For this review, take the finished solid that the model builds, in its own axes (mm). A direction names the side the tool comes from. Round coordinates to 2 decimals unless told otherwise and drop trailing zeros. Loops run counter-clockwise (first coordinate to the right, second up) from the corner with the lowest first, then second, coordinate; pieces in that order, holes last. Notation, with made-up numbers: M -27.5,66 L 21.5,66 A9 cw 21.5,78 Z; hole C -19.75,86 d8. An arc over 180 degrees is marked long. One line per question, with ' | ' between items. Start each with the question number.
1) Mouldability with a two-part tool opening along Y and no side actions: class faces 3 (the face through (-97.62, -0.75, -175.27)), 4 (the face through (-55, -16, -74)), 5 (the face through (-66.373, -7.923, -79.231)) as pulls with the +Y half, pulls with the -Y half, needs draft (parallel to the pull), parting line crosses it, or undercut.
2) For pin 1 Ø4 at (y, z) = (-8.5, -84) entering from +X; pin 2 Ø1 at (x, y) = (-48, -14) entering from -Z; pin 3 Ø8 at (x, y) = (3, -5.5) entering from -Z; pin 4 Ø3 at (x, z) = (0, 0) entering from +Y, all flat-tipped, find the tip position at first contact; note any pin that passes through.
3) For probe 1 along Y at (x, z) = (10.5, 0.5); probe 2 along X at (y, z) = (-2, -0.5); probe 3 along X at (y, z) = (-12, 5), list the stretches that pass through material, from the lowest coordinate up. Write a range as from..to.
4) For faces 1 (the face through (-58.322, -7.923, -101.605)), 2 (the face through (0, -8, -3)), list the 3-axis set-ups (+Z, -Z, +X, -X, +Y, -Y) from which the entire face can be reached by the end or side of a thin tool; tool diameter is ignored.
5) We need section A-A (y = -10.5). Give the boundary of the cut face in (x, z), and give its area (3 significant figures).
```python
from build123d import *

# Parameters (mm, degrees)
F1_DEPTH     = 16
F2_DEPTH     = 8
F3_T1_DEPTH  = 28.5
F3_T3_DEPTH  = 176.25
F3_T5_DEPTH  = 206.25
F3_T8_ANGLE  = 113.8828315396
F3_T10_ANGLE = 205.3052563157
F3_T12_ANGLE = 301.0526480562
F3_T14_ANGLE = 87.1421031631
F3_T16_ANGLE = 90
F3_T18_ANGLE = 202.4999999088
F3_T20_ANGLE = 256.2183340246
F3_T22_ANGLE = 87.1421031631
F4_D         = 5


# Not quite as in the source:
# - a fillet or chamfer that OpenCascade refuses, or shapes differently, is made with other operations: its cross-section is extruded or revolved along the edge and cut away or added


with BuildPart() as f1:
    # F0 (on Front) → F1 (new body)
    with BuildSketch(Plane.XZ):
        Polygon((-25.3386959586, -21.9761344899), (-13.8581929877, 5.7402514855), (-28.6402655078, 11.8631864033), (-105.1769519809, -172.9127200989), (-90.3948794607, -179.0356550168), align=None)
        with BuildLine():
            Line((-28.6402655078, 11.8631864033), (-13.8581929877, 5.7402514855))
            ThreePointArc((-13.8581929877, 5.7402514855), (-8.3335534854, 12.4720441912), (2.39e-08, 15))
            ThreePointArc((2.39e-08, 15), (-8, 22.9999999881), (0, 31))
            ThreePointArc((0, 31), (-17.2226772236, 25.7755579814), (-28.6402655078, 11.8631864033))
        make_face()
        with BuildLine():
            ThreePointArc((-5.7402514855, -13.8581929877), (-13.8581929877, -5.7402514855), (-13.8581929877, 5.7402514855))
            Line((-13.8581929877, 5.7402514855), (-25.3386959586, -21.9761344899))
            ThreePointArc((-25.3386959586, -21.9761344899), (-17.2207544564, -13.8581929877), (-5.7402514855, -13.8581929877))
        make_face()
    extrude(amount=F1_DEPTH)

    # F0 (on Front) → F2 (join)
    with BuildSketch(Plane.XZ):
        with BuildLine():
            Line((0, 0), (-13.8581929877, 5.7402514855))
            ThreePointArc((-13.8581929877, 5.7402514855), (-13.8581929877, -5.7402514855), (-5.7402514855, -13.8581929877))
            Line((-5.7402514855, -13.8581929877), (0, 0))
        make_face()
        with BuildLine():
            ThreePointArc((2.39e-08, 15), (-8.3335534854, 12.4720441912), (-13.8581929877, 5.7402514855))
            Line((-13.8581929877, 5.7402514855), (0, 0))
            Line((0, 0), (-5.7402514855, -13.8581929877))
            ThreePointArc((-5.7402514855, -13.8581929877), (8.3335534953, -12.4720441845), (15, 0))
            ThreePointArc((15, 0), (10.6066017262, 10.6066017094), (2.39e-08, 15))
        make_face()
    extrude(amount=F2_DEPTH)

    # F3: fillet of radius 2.5 on 14 edges, made by hand

    # F3_s2 → F3_t1 (cut)
    with BuildSketch(Plane(origin=(-34.414512586, 0, 14.2549578556), x_dir=(0, 1, 0), z_dir=(0.9238795325, 0, -0.3826834324))):
        with BuildLine():
            ThreePointArc((-13.5, -200), (-15.267766953, -199.267766953), (-16, -197.5))
            Line((-16, -197.5), (-16, -200))
            Line((-16, -200), (-13.5, -200))
        make_face()
        with BuildLine():
            ThreePointArc((-2.5, -200), (-0.732233047, -199.267766953), (0, -197.5))
            Line((0, -197.5), (0, -200))
            Line((0, -200), (-2.5, -200))
        make_face()
    extrude(amount=F3_T1_DEPTH, mode=Mode.SUBTRACT)

    # F3_s4 → F3_t3 (cut)
    with BuildSketch(Plane(origin=(-78.9284579253, 0, -190.5501535805), x_dir=(0, 1, 0), z_dir=(0.3826834324, 0, 0.9238795325))):
        with BuildLine():
            ThreePointArc((-13.5, 15), (-15.267766953, 15.732233047), (-16, 17.5))
            Line((-16, 17.5), (-16, 15))
            Line((-16, 15), (-13.5, 15))
        make_face()
        with BuildLine():
            ThreePointArc((-2.5, 15), (-0.732233047, 15.732233047), (0, 17.5))
            Line((0, 17.5), (0, 15))
            Line((0, 15), (-2.5, 15))
        make_face()
    extrude(amount=F3_T3_DEPTH, mode=Mode.SUBTRACT)

    # F3_s6 → F3_t5 (cut)
    with BuildSketch(Plane(origin=(0, 0, 0), x_dir=(0, 1, 0), z_dir=(-0.3826834324, 0, -0.9238795325))):
        with BuildLine():
            ThreePointArc((-13.5, -31), (-15.267766953, -30.267766953), (-16, -28.5))
            Line((-16, -28.5), (-16, -31))
            Line((-16, -31), (-13.5, -31))
        make_face()
        with BuildLine():
            ThreePointArc((-2.5, -31), (-0.732233047, -30.267766953), (0, -28.5))
            Line((0, -28.5), (0, -31))
            Line((0, -31), (-2.5, -31))
        make_face()
    extrude(amount=F3_T5_DEPTH, mode=Mode.SUBTRACT)

    # F3_s7 → F3_t8 (revolve, cut)
    with BuildSketch(Plane(origin=(-11.480502971, 0, -27.7163859753), x_dir=(0, 1, 0), z_dir=(-0.3826834324, 0, -0.9238795325))):
        with BuildLine():
            ThreePointArc((-16, -17.5), (-15.267766953, -15.732233047), (-13.5, -15))
            Line((-13.5, -15), (-16, -15))
            Line((-16, -15), (-16, -17.5))
        make_face()
    revolve(axis=Axis((-11.480502971, -16, -27.7163859753), (0, 1, 0)), revolution_arc=F3_T8_ANGLE, mode=Mode.SUBTRACT)

    # F3_s9 → F3_t10 (revolve, cut)
    with BuildSketch(Plane(origin=(0, 0, 0), x_dir=(0, 1, 0), z_dir=(0.999700368, 0, 0.0244780336))):
        with BuildLine():
            ThreePointArc((-16, -17.5), (-15.267766953, -15.732233047), (-13.5, -15))
            Line((-13.5, -15), (-16, -15))
            Line((-16, -15), (-16, -17.5))
        make_face()
    revolve(axis=Axis((0, -16, 0), (0, 1, 0)), revolution_arc=F3_T10_ANGLE, mode=Mode.SUBTRACT)

    # F3_s11 → F3_t12 (revolve, cut)
    with BuildSketch(Plane(origin=(11.4998076678, 0, 11.4334898289), x_dir=(0, 1, 0), z_dir=(0.7091486068, 0, 0.7050590425))):
        with BuildLine():
            ThreePointArc((-16, 5.8104179571), (-15.267766953, 7.5781849101), (-13.5, 8.3104179571))
            Line((-13.5, 8.3104179571), (-16, 8.3104179571))
            Line((-16, 8.3104179571), (-16, 5.8104179571))
        make_face()
    revolve(axis=Axis((0, -16, 23), (0, 1, 0)), revolution_arc=F3_T12_ANGLE, mode=Mode.SUBTRACT)

    # F3_s13 → F3_t14 (revolve, cut)
    with BuildSketch(Plane(origin=(0, 0, 0), x_dir=(0, 1, 0), z_dir=(0.9418106956, 0, -0.3361437395))):
        with BuildLine():
            ThreePointArc((-16, 28.5), (-15.267766953, 30.267766953), (-13.5, 31))
            Line((-13.5, 31), (-16, 31))
            Line((-16, 31), (-16, 28.5))
        make_face()
    revolve(axis=Axis((0, -16, 0), (0, -1, 0)), revolution_arc=F3_T14_ANGLE, mode=Mode.SUBTRACT)

    # F3_s15 → F3_t16 (revolve, cut)
    with BuildSketch(Plane(origin=(-11.480502971, 0, -27.7163859753), x_dir=(0, 1, 0), z_dir=(-0.3826834324, 0, -0.9238795325))):
        with BuildLine():
            ThreePointArc((0, -17.5), (-0.732233047, -15.732233047), (-2.5, -15))
            Line((-2.5, -15), (0, -15))
            Line((0, -15), (0, -17.5))
        make_face()
    revolve(axis=Axis((-11.480502971, 0, -27.7163859753), (0, 1, 0)), revolution_arc=F3_T16_ANGLE, mode=Mode.SUBTRACT)

    # F3_s17 → F3_t18 (revolve, cut)
    with BuildSketch(Plane(origin=(0, 0, 0), x_dir=(0, 1, 0), z_dir=(-0.9238795325, 0, 0.3826834324))):
        with BuildLine():
            ThreePointArc((0, 12.5), (-0.732233047, 14.267766953), (-2.5, 15))
            Line((-2.5, 15), (0, 15))
            Line((0, 15), (0, 12.5))
        make_face()
    revolve(axis=Axis((0, 0, 0), (0, -1, 0)), revolution_arc=F3_T18_ANGLE, mode=Mode.SUBTRACT)

    # F3_s19 → F3_t20 (revolve, cut)
    with BuildSketch(Plane.YZ):
        with BuildLine():
            ThreePointArc((0, 12.5), (-0.732233047, 14.267766953), (-2.5, 15))
            Line((-2.5, 15), (0, 15))
            Line((0, 15), (0, 12.5))
        make_face()
    revolve(axis=Axis((0, 0, 23), (0, 1, 0)), revolution_arc=F3_T20_ANGLE, mode=Mode.SUBTRACT)

    # F3_s21 → F3_t22 (revolve, cut)
    with BuildSketch(Plane(origin=(0, 0, 0), x_dir=(0, 1, 0), z_dir=(0.9418106956, 0, -0.3361437395))):
        with BuildLine():
            ThreePointArc((0, 28.5), (-0.732233047, 30.267766953), (-2.5, 31))
            Line((-2.5, 31), (0, 31))
            Line((0, 31), (0, 28.5))
        make_face()
    revolve(axis=Axis((0, 0, 0), (0, -1, 0)), revolution_arc=F3_T22_ANGLE, mode=Mode.SUBTRACT)

    # F4 (through all)
    with Locations(Plane(origin=(0, 0, 0), x_dir=(1, 0, 0), z_dir=(0, 1, 0))):
        with Locations((0, 0)):
            Hole(F4_D / 2)


solid = f1.part
```
Answers below:
1) face 3: pulls with the +Y half | face 4: pulls with the -Y half | face 5: needs draft
2) pin 1: x = -50.2 | pin 2: z = -77.78 | pin 3: z = -15 | pin 4: through
3) probe 1: -8..0 | probe 2: -33.71..-2.45, 2.45..14.94 | probe 3: -31.48..-14.14
4) face 1: -Z, +X, +Y, -Y | face 2: +X, -Y
5) outline: M -105.18,-172.91 L -90.39,-179.04 L -25.34,-21.98 A15 cw -5.74,-13.86 A15 cw 0,15 A8 cw 0,31 A31 ccw -28.64,11.86 Z | area: 3,630 mm^2
